The listing builds one solid part. Answer for the finished solid, in the listing's coordinates (mm). Face numbers are marked on the shaded views. A direction names the side the tool comes from. Coordinates: 2 decimals unless noted, no trailing zeros. Write each loop counter-clockwise with the first axis right and the second up, starting at its lowest first coordinate (ties: lowest second). Pieces come first, ordered by that corner, then holes. Notation, with made-up numbers: M -14.75,45.25 L 44.25,45.25 A19 ccw 44.25,80.25 Z; hole C -29.75,85.25 d9. An arc over 180 degrees is marked long. Answer as CSV lines item,"result".
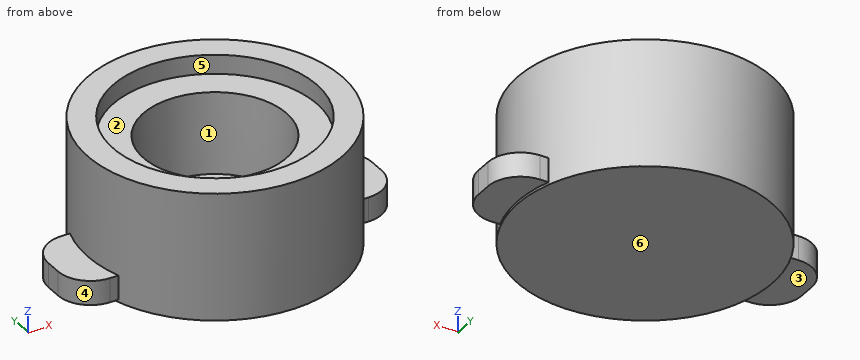
```python
from build123d import *

# Parameters (mm, degrees)
F0_R     = 20
F1_DEPTH = 20
F2_R     = 16
F3_DEPTH = 3
F4_R     = 11.25
F5_DEPTH = 12.5
F5_TAPER = 3
F6_W     = 12.7
F6_H     = 3.81
F7_DEPTH = 25.4
F8_DEPTH = 25.4
F9_R     = 5.08


with BuildPart() as f1:
    # F0 (on Top) → F1 (new body)
    with BuildSketch(Plane.XY):
        Circle(F0_R)
    extrude(amount=-F1_DEPTH)

    # F2 (on face) → F3 (cut)
    with BuildSketch(Plane.XY):
        Circle(F2_R)
    extrude(amount=-F3_DEPTH, mode=Mode.SUBTRACT)

    # F4 (on face) → F5 (cut)
    with BuildSketch(Plane.XY.offset(-3)):
        Circle(F4_R)
    extrude(amount=-F5_DEPTH, taper=F5_TAPER, mode=Mode.SUBTRACT)

    # F6 (on Right) → F7 (join)
    with BuildSketch(Plane.YZ):
        with Locations((0, -17.6945884627)):
            Rectangle(F6_W, F6_H)
    extrude(amount=F7_DEPTH)

    # F6 (on Right) → F8 (join)
    with BuildSketch(Plane.YZ):
        with Locations((0, -17.6945884627)):
            Rectangle(F6_W, F6_H)
    extrude(amount=-F8_DEPTH)

    # F9
    f9_edges = [f1.edges().sort_by_distance(p)[0] for p in [
        (-25.4, 6.35, -17.694588),
        (-25.4, -6.35, -17.694588),
        (25.4, -6.35, -17.694588),
        (25.4, 6.35, -17.694588),
    ]]
    fillet(f9_edges, radius=F9_R)


solid = f1.part
```
Q1. Find section C-C (z = -7). Give the vertices of the cut face in (x, y), and give its area (3 significant figures).
Output:
outline,"C 0,0 d40; hole C 0,0 d22.08"
area,"874 mm2"
Q2. The mould has two halves that part along Y. Classify the marked faces 1, 2, 3 and 4: pulls with the +Y half, pulls with the -Y half, needs draft (parallel to the pull), parting line crosses it, or undercut.
Output:
face 1,"undercut"
face 2,"undercut"
face 3,"needs draft"
face 4,"pulls with the -Y half"
Q3. Find section D-D (x = 12.5). Give the vertices of the cut face in (y, z).
Output:
outline,"M -15.61,-20 L 15.61,-20 L 15.61,0 L 9.99,0 L 9.99,-3 L -9.99,-3 L -9.99,0 L -15.61,0 Z"
Q4. For the marked faces 5 and 6, determine the directions among +Z, -Z, +X, -X, +Y, -Y from which every point of the face is accessible in a straight line to the end or side of a thin tool.
Output:
face 5,"+Z"
face 6,"-Z, +X, -X, +Y, -Y"
Q5. Flat-ended cylindrical pins translate along their axes: pin 1 Ø10 at (y, z) = (-6, -12.5) entering from -X; pin 2 Ø1 at (y, z) = (-12, -17.5) entering from +X; pin 3 Ø0.7 at (x, z) = (-19.5, -18) entering from -Y. Find the tip coordinate at first contact, or state that the pin passes through.
Output:
pin 1,"x = -25.31"
pin 2,"x = 16.36"
pin 3,"y = -6.35"
Q6. Find section B-B (y = -14). Give the vertices of the cut face in (x, z).
Output:
outline,"M -14.28,-20 L 14.28,-20 L 14.28,0 L 7.75,0 L 7.75,-3 L -7.75,-3 L -7.75,0 L -14.28,0 Z"
Q7. Straight lines are drawn through the part: line 1 (Y direction, x = 0, z = -1.1); line 2 (Y direction, x = -12, z = -14.5); line 3 (Z direction, x = -3, y = 3). For each, find the intervals that lie inside material, in ascending order.
Output:
line 1,"-20 to -16, 16 to 20"
line 2,"-16 to 16"
line 3,"-20 to -15.5"
Q8. Find section A-A (x = 0). Give the vertices of the cut face in (y, z).
Output:
outline,"M -20,-20 L 20,-20 L 20,0 L 16,0 L 16,-3 L 11.25,-3 L 10.59,-15.5 L -10.59,-15.5 L -11.25,-3 L -16,-3 L -16,0 L -20,0 Z"
